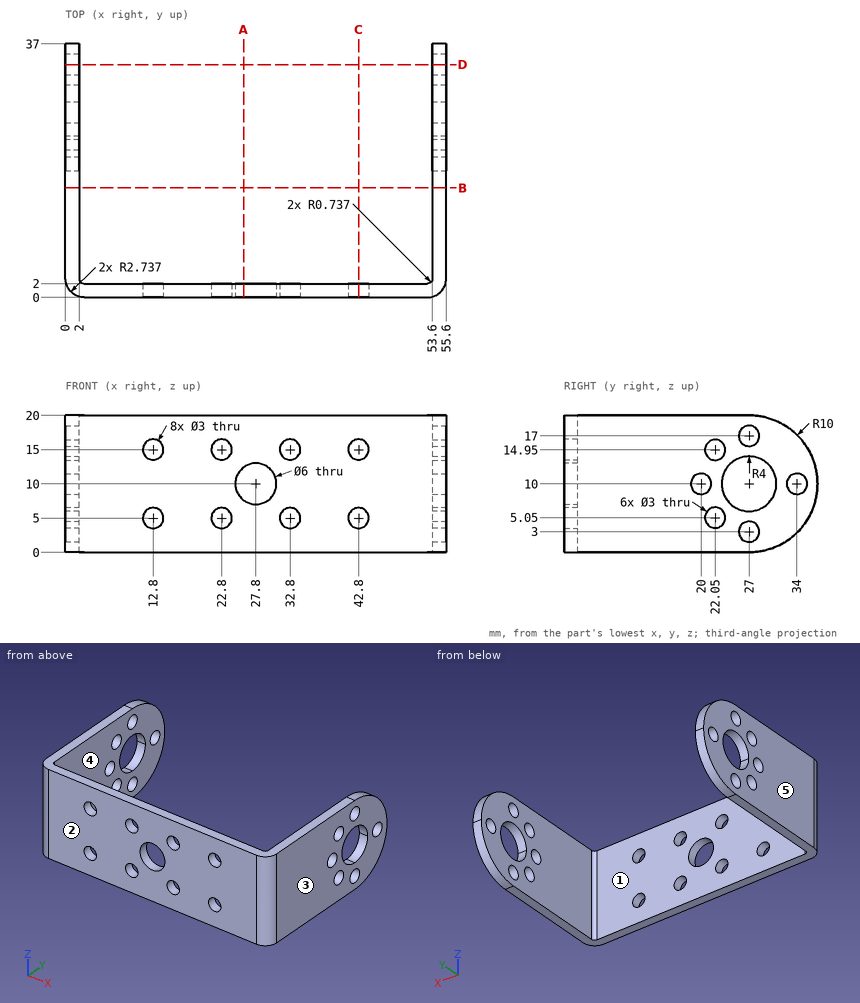
Answer from the drawing. Dimensions are ordinates in mm from the lowest x, y and z of the part. A direction names the side the tool comes from. Give positions to 0.01 mm unless a question says otherwise; leave off trailing zeros. Loops run counter-clockwise (first coordinate to the right, second up) from the corner with the lowest first, then second, coordinate; pieces in that order, holes last. Notation, with made-up numbers: M 23,78.5 L 59,78.5 A28 ccw 59,99.5 Z; hole C 81,-11.75 d4. An arc over 180 degrees is marked long. One line per item, written item: value.
Q1. A cutting plane is placed at D-D on y = 34. Determine the outline of the cut face in (x, z).
Working result:
outline: M 0,2.86 L 2,2.86 L 2,8.5 L 0,8.5 Z; M 0,11.5 L 2,11.5 L 2,17.14 L 0,17.14 Z; M 53.6,2.86 L 55.6,2.86 L 55.6,8.5 L 53.6,8.5 Z; M 53.6,11.5 L 55.6,11.5 L 55.6,17.14 L 53.6,17.14 Z
Q2. A cutting plane is placed at B-B on y = 16. Determine the outline of the cut face in (x, z).
Working result:
outline: M 0,0 L 2,0 L 2,20 L 0,20 Z; M 53.6,0 L 55.6,0 L 55.6,20 L 53.6,20 Z
Q3. A cutting plane is placed at A-A on x = 26. Determine the outline of the cut face in (y, z).
Working result:
outline: M 0,0 L 2,0 L 2,7.6 L 0,7.6 Z; M 0,12.4 L 2,12.4 L 2,20 L 0,20 Z
Q4. A flat-ended cylindrical pin translates along its axis: P1, Ø1, axis at x = 18, z = 3.5, coming from the +Y side. Find the tip coordinate at first contact, or state that the pin passes through.
Working result:
P1: stops at y = 2
Q5. A cutting plane is placed at C-C on x = 42.8. Determine the outline of the cut face in (y, z), then the cut area to 3 significant figures.
Working result:
outline: M 0,0 L 2,0 L 2,3.5 L 0,3.5 Z; M 0,6.5 L 2,6.5 L 2,13.5 L 0,13.5 Z; M 0,16.5 L 2,16.5 L 2,20 L 0,20 Z
area: 28.0 mm^2
Q6. Find the intervals of material crossed by line 1 (X direction, y = 0.9, z = 15); line 2 (X direction, y = 14.5, z = 5.5); line 3 (Z direction, x = 22, y = 1), in increasing order. Write a range as from..to.
Working result:
line 1: x = 0.71..11.3, 14.3..21.3, 24.3..31.3, 34.3..41.3, 44.3..54.89
line 2: x = 0..2, 53.6..55.6
line 3: z = 0..3.73, 6.27..13.73, 16.27..20
Q7. Determine the mould class of the marked faces 3, 4 and 5 for opening direction X: +X half, -X half, draft (parallel to the pull), parting line (faces both ways), or undercut.
Working result:
face 3: +X half
face 4: undercut
face 5: -X half
Q8. For the marked faces 1 and 2, determine the directions among +Z, -Z, +X, -X, +Y, -Y from which every point of the face is accessible in a straight line to the end or side of a thin tool.
Working result:
face 1: +Z, -Z, +Y
face 2: +Z, -Z, +X, -X, -Y
